Read the model definition and answer for the solid it produces. Units are mm, in the model's axes. A direction names the side the tool comes from. Coordinates: 2 decimals unless noted, no trailing zeros. Write each loop counter-clockwise with the first axis right and the second up, starting at its lowest first coordinate (ties: lowest second). Pieces come first, ordered by that corner, then holes. Notation, with made-up numbers: (33.25, -31) - (77.25, -31) arc R15 cw to (77.25, -13) - close; hole circle Ø4 at (11.5, -22.75). An arc over 180 degrees is marked (long way). Use a Markdown table: item, result.
from build123d import *

# Parameters (mm, degrees)
F1_DEPTH     = 114
F3_DEPTH     = 3
F5_R         = 0.5
F6_D         = 5.2
F6_DEPTH     = 231.001
F7_D         = 5.2
F8_T1_DEPTH  = 12
F8_T6_ANGLE  = 161.6484946187
F8_T11_ANGLE = 150.9012204259
F8_T16_ANGLE = 150.9012204259
F8_T21_ANGLE = 161.6484946187


# Not quite as in the source:
# - a fillet or chamfer that OpenCascade refuses, or shapes differently, is made with other operations: its cross-section is extruded or revolved along the edge and cut away or added


with BuildPart() as f1:
    # F0 (on Right) → F1 (new body, symmetric)
    with BuildSketch(Plane.YZ):
        with BuildLine():
            Line((2.5, 5), (-9.5, 5))
            ThreePointArc((-9.5, 5), (-10.9142135624, 4.4142135624), (-11.5, 3))
            Line((-11.5, 3), (-11.5, 0))
            Line((-11.5, 0), (0, 0))
            Line((0, 0), (3.5, 0))
            Line((3.5, 0), (3.5, 4))
            ThreePointArc((3.5, 4), (3.2071067812, 4.7071067812), (2.5, 5))
        make_face()
        with BuildLine():
            Line((3.5, -6), (3.5, 0))
            Line((3.5, 0), (0, 0))
            Line((0, 0), (0, -5))
            ThreePointArc((0, -5), (0.5857864376, -6.4142135624), (2, -7))
            Line((2, -7), (2.5, -7))
            ThreePointArc((2.5, -7), (3.2071067812, -6.7071067812), (3.5, -6))
        make_face()
    extrude(amount=F1_DEPTH, both=True)

    # F2 (on face) → F3 (join)
    with BuildSketch(Plane.YZ.offset(114)):
        with BuildLine():
            Line((2.5, 28.5), (-24.5, 28.5))
            ThreePointArc((-24.5, 28.5), (-28.7426406871, 26.7426406871), (-30.5, 22.5))
            Line((-30.5, 22.5), (-30.5, 12.5))
            ThreePointArc((-30.5, 12.5), (-29.0355339059, 8.9644660941), (-25.5, 7.5))
            Line((-25.5, 7.5), (-13.5, 7.5))
            ThreePointArc((-13.5, 7.5), (-12.0857864376, 6.9142135624), (-11.5, 5.5))
            Line((-11.5, 5.5), (-11.5, 0))
            Line((-11.5, 0), (0, 0))
            Line((0, 0), (0, -6))
            ThreePointArc((0, -6), (0.2928932188, -6.7071067812), (1, -7))
            Line((1, -7), (2.5, -7))
            ThreePointArc((2.5, -7), (3.2071067812, -6.7071067812), (3.5, -6))
            Line((3.5, -6), (3.5, 7.5))
            Line((3.5, 7.5), (3.5, 27.5))
            ThreePointArc((3.5, 27.5), (3.2071067812, 28.2071067812), (2.5, 28.5))
        make_face()
    extrude(amount=F3_DEPTH)

    # F4: F1 across plane


with BuildPart() as f1_1:
    add(f1.part)
    add(f1.part.mirror(Plane.YZ))

    # F5
    f5_edges = [f1_1.edges().sort_by_distance(p)[0] for p in [
        (0, 0, 0),
    ]]
    fillet(f5_edges, radius=F5_R)

    # F6 (through all, one way)
    with BuildSketch(Plane.YZ.offset(114)):
        with Locations((-24.5, 18)):
            Circle(F6_D / 2)
    extrude(amount=-F6_DEPTH, mode=Mode.SUBTRACT)

    # F7 (through all)
    with Locations(Plane(origin=(114, 0, 0), x_dir=(0, 1, 0), z_dir=(-1, 0, 0))):
        with Locations((-24.5, -18)):
            Hole(F7_D / 2)

    # F8: fillet of radius 0.5 on 6 edges, made by hand

    # F8_s2 → F8_t1 (join)
    with BuildSketch(Plane.XZ.offset(-2.5)):
        with BuildLine():
            ThreePointArc((-114, 5.5), (-113.8535533906, 5.1464466094), (-113.5, 5))
            Line((-113.5, 5), (-114, 5))
            Line((-114, 5), (-114, 5.5))
        make_face()
        with BuildLine():
            ThreePointArc((114, 5.5), (113.8535533906, 5.1464466094), (113.5, 5))
            Line((113.5, 5), (114, 5))
            Line((114, 5), (114, 5.5))
        make_face()
    extrude(amount=F8_T1_DEPTH)


with BuildPart() as f8_tool4:
    # F8_s5 → F8_t6 (revolve)
    with BuildSketch(Plane(origin=(0, 3.4475148544, 1.1435956184), x_dir=(1, 0, 0), z_dir=(0, -0.9491428342, -0.3148458041))):
        with BuildLine():
            ThreePointArc((-114, 1.5094568264), (-113.8535533906, 1.863010217), (-113.5, 2.0094568264))
            Line((-113.5, 2.0094568264), (-114, 2.0094568264))
            Line((-114, 2.0094568264), (-114, 1.5094568264))
        make_face()
    revolve(axis=Axis((-114, 2.5, 4), (1, 0, 0)), revolution_arc=F8_T6_ANGLE)

    split(bisect_by=Plane.XZ.offset(-3.5), keep=Keep.TOP)


with BuildPart() as f1_2:
    add(f1_1.part)

    # F8_t3: union F8_tool4
    add(f8_tool4.part)


with BuildPart() as f8_tool9:
    # F8_s10 → F8_t11 (revolve)
    with BuildSketch(Plane.XZ.offset(9.5)):
        with BuildLine():
            ThreePointArc((-114, 5.5), (-113.8535533906, 5.1464466094), (-113.5, 5))
            Line((-113.5, 5), (-114, 5))
            Line((-114, 5), (-114, 5.5))
        make_face()
    revolve(axis=Axis((-114, -9.5, 3), (1, 0, 0)), revolution_arc=F8_T11_ANGLE)

    split(bisect_by=Plane.XZ.offset(11.5), keep=Keep.BOTTOM)


with BuildPart() as f1_3:
    add(f1_2.part)

    # F8_t8: union F8_tool9
    add(f8_tool9.part)


with BuildPart() as f8_tool14:
    # F8_s15 → F8_t16 (revolve)
    with BuildSketch(Plane.XZ.offset(9.5)):
        with BuildLine():
            ThreePointArc((113.5, 5), (113.8535533906, 5.1464466094), (114, 5.5))
            Line((114, 5.5), (114, 5))
            Line((114, 5), (113.5, 5))
        make_face()
    revolve(axis=Axis((114, -9.5, 3), (1, 0, 0)), revolution_arc=F8_T16_ANGLE)

    split(bisect_by=Plane.XZ.offset(11.5), keep=Keep.BOTTOM)


with BuildPart() as f1_4:
    add(f1_3.part)

    # F8_t13: union F8_tool14
    add(f8_tool14.part)


with BuildPart() as f8_tool19:
    # F8_s20 → F8_t21 (revolve)
    with BuildSketch(Plane(origin=(0, 3.4475148544, 1.1435956184), x_dir=(1, 0, 0), z_dir=(0, -0.9491428342, -0.3148458041))):
        with BuildLine():
            ThreePointArc((114, 1.5094568264), (113.8535533906, 1.863010217), (113.5, 2.0094568264))
            Line((113.5, 2.0094568264), (114, 2.0094568264))
            Line((114, 2.0094568264), (114, 1.5094568264))
        make_face()
    revolve(axis=Axis((114, 2.5, 4), (1, 0, 0)), revolution_arc=F8_T21_ANGLE)

    split(bisect_by=Plane.XZ.offset(-3.5), keep=Keep.TOP)


with BuildPart() as f1_5:
    add(f1_4.part)

    # F8_t18: union F8_tool19
    add(f8_tool19.part)


solid = f1_5.part
(1) A cutting plane is placed at A-A, the plane z = 18. Write down the section's boundary in (x, y), and give its area (3 significant figures).
Report:
| item | result |
|---|---|
| outline | (-117, -30.5) - (-114, -30.5) - (-114, -27.1) - (-117, -27.1) - close; (-117, -21.9) - (-114, -21.9) - (-114, 3.5) - (-117, 3.5) - close; (114, -30.5) - (117, -30.5) - (117, -27.1) - (114, -27.1) - close; (114, -21.9) - (117, -21.9) - (117, 3.5) - (114, 3.5) - close |
| area | 173 mm² |
(2) A cutting plane is placed at B-B, the plane x = 91.5. Write down the section's boundary in (y, z), and give its area (3 significant figures).
Report:
| item | result |
|---|---|
| outline | (-11.5, 0) - (-0.5, 0) arc R0.5 cw to (0, -0.5) - (0, -5) arc R2 ccw to (2, -7) - (2.5, -7) arc R1 ccw to (3.5, -6) - (3.5, 4) arc R1 ccw to (2.5, 5) - (-9.5, 5) arc R2 ccw to (-11.5, 3) - close |
| area | 97.4 mm² |
(3) Each of these flat-tipped pins is pushed along its axis until it touches: P1, Ø1.7, axis at x = 40, z = 3.5, coming from the -Y side; P2, Ø1.5, axis at x = 115.5, y = -19.5, coming from the -Z side; P3, Ø10, axis at x = 1.5, y = -3.5, coming from the +Z side. Where does it stop, or does it pass through?
Report:
| item | result |
|---|---|
| P1 | stops at y = -11.5 |
| P2 | stops at z = 7.5 |
| P3 | stops at z = 5 |
(4) Straight lines are drawn through the part: L1, parallel to Z at x = -115.55, y = -24.5; L2, parallel to X at y = -3, z = 7.5; L3, parallel to Y at x = 115.45, z = 18. For each, find the intervals that lie inside material, in ascending order.
Report:
| item | result |
|---|---|
| L1 | z = 7.5 to 15.4, 20.6 to 28.5 |
| L2 | x = -117 to -114, 114 to 117 |
| L3 | y = -30.5 to -27.1, -21.9 to 3.5 |
(5) For faces 1 (the flat face through (1, 3.5, -2)), 2 (the flat face through (2, -6, 0)), 3 (the flat face through (2, -3, 5)), determine the directions among +Z, -Z, +X, -X, +Y, -Y from which every point of the face is accessible in a straight line to the end or side of a thin tool.
Report:
| item | result |
|---|---|
| face 1 | +Z, -Z, +X, -X, +Y |
| face 2 | -Z, +X, -X, -Y |
| face 3 | +Z, +Y, -Y |
(6) The mould has two halves that part along X. Classify faces 4 (the flat face through (117, -10, 15)), 5 (the flat face through (-114, -14, 17)), 6 (the flat face through (2, 0, -3)): pulls with the +X half, pulls with the -X half, needs draft (parallel to the pull), parting line crosses it, or undercut.
Report:
| item | result |
|---|---|
| face 4 | pulls with the +X half |
| face 5 | undercut |
| face 6 | needs draft |
